Here's how the part is built. I have some questions about the finished solid (model axes, mm). Give positions to 0.01 mm unless a question says otherwise; leave off trailing zeros. Write each loop counter-clockwise with the first axis right and the second up, starting at its lowest first coordinate (ties: lowest second). Pieces come first, ordered by that corner, then holes. Notation, with made-up numbers: (3, 81) - (61, 81) arc R14 cw to (61, 99) - close; hole circle Ø2 at (78, -34). An arc over 180 degrees is marked (long way). Write each question's results on one line, items separated by ' | '. Start each with the question number.
Item 1: Will these pins go through, and if not, where does the flat tip stop? P1, Ø1, axis at y = 0.5, z = -83.5, coming from the +X side; P2, Ø1.6, axis at x = 12.5, y = -0.5, coming from the -Z side; P3, Ø1, axis at y = 0.5, z = -85, coming from the -X side.
Item 2: Please list where this line runs through material, in increasing order: line 1 along Z through (x, y) = (-26, -1.4).
Item 3: Suppose I cut it at A-A on x = 1.5. List the corners of the cut face in (y, z) for me.
```python
from build123d import *

# Parameters (mm, degrees)
SKETCH1_W           = 635.3556
SKETCH1_H           = 165.1
BOSS_EXTRUDE1_DEPTH = 1.5875
SKETCH2_W           = 254
SKETCH2_H           = 3.175
BOSS_EXTRUDE2_DEPTH = 3.175


with BuildPart() as part:
    # Sketch1 → Boss-Extrude1 (new, symmetric)
    with BuildSketch(Plane(origin=(0, 0, 0), x_dir=(1, 0, 0), z_dir=(0, 1, 0))):
        Rectangle(SKETCH1_W, SKETCH1_H)
    extrude(amount=BOSS_EXTRUDE1_DEPTH, both=True)

    # Sketch2 → Boss-Extrude2 (add)
    with BuildSketch(Plane(origin=(0, 0, -82.55), x_dir=(-1, 0, 0), z_dir=(0, 0, -1))):
        with Locations((-157.8229, 0)):
            Rectangle(SKETCH2_W, SKETCH2_H)
        with Locations((157.8229, 0)):
            Rectangle(SKETCH2_W, SKETCH2_H)
    extrude(amount=BOSS_EXTRUDE2_DEPTH)


solid = part.part
```
Checked values:
1) P1: stops at x = 284.82 | P2: stops at z = -82.55 | P3: stops at x = -284.82
2) line 1: z = -82.55 to 82.55
3) outline: (-1.59, -82.55) - (1.59, -82.55) - (1.59, 82.55) - (-1.59, 82.55) - close
